Can you work these out from the model? Positions are in its coordinate system, mm. Give positions to 0.01 mm unless a question says otherwise; leave off trailing zeros. Write each loop counter-clockwise with the first axis right and the second up, starting at its lowest first coordinate (ties: lowest second). Pieces come first, ordered by that corner, then holes.
from build123d import *

# Parameters (mm, degrees)
SKETCH1_W               = 56
SKETCH1_H               = 56
SKETCH1_R               = 1.5
SKETCH1_W_2             = 46
SKETCH1_H_2             = 46
BOSS_EXTRUDE1_DEPTH     = 6
BOSS_EXTRUDE2_START     = 6
SKETCH1_2_W             = 56
SKETCH1_2_H             = 56
SKETCH1_2_R             = 1.5
BOSS_EXTRUDE2_DEPTH     = 2
CUT_EXTRUDE1_DEPTH      = 7
CUT_EXTRUDE1_DEPTH_BACK = 3
FILLET1_R               = 2


with BuildPart() as part:
    # Sketch1 → Boss-Extrude1 (new body)
    with BuildSketch(Plane(origin=(0, 0, 0), x_dir=(1, 0, 0), z_dir=(0, 1, 0))):
        Rectangle(SKETCH1_W, SKETCH1_H)
        with Locations((-25, 25)):
            Circle(SKETCH1_R, mode=Mode.SUBTRACT)
        with Locations((25, 25)):
            Circle(SKETCH1_R, mode=Mode.SUBTRACT)
        with Locations((25, -25)):
            Circle(SKETCH1_R, mode=Mode.SUBTRACT)
        with Locations((-25, -25)):
            Circle(SKETCH1_R, mode=Mode.SUBTRACT)
        Rectangle(SKETCH1_W_2, SKETCH1_H_2, mode=Mode.SUBTRACT)
    extrude(amount=BOSS_EXTRUDE1_DEPTH)

    # Sketch1<2> → Boss-Extrude2 (add)
    with BuildSketch(Plane(origin=(0, 0, 0), x_dir=(1, 0, 0), z_dir=(0, 1, 0)).offset(BOSS_EXTRUDE2_START)):
        Rectangle(SKETCH1_2_W, SKETCH1_2_H)
        with Locations((-25, 25)):
            Circle(SKETCH1_2_R, mode=Mode.SUBTRACT)
        with Locations((25, 25)):
            Circle(SKETCH1_2_R, mode=Mode.SUBTRACT)
        with Locations((25, -25)):
            Circle(SKETCH1_2_R, mode=Mode.SUBTRACT)
        with Locations((-25, -25)):
            Circle(SKETCH1_2_R, mode=Mode.SUBTRACT)
    extrude(amount=BOSS_EXTRUDE2_DEPTH)

    # Sketch2 → Cut-Extrude1 (cut, two sides)
    with BuildSketch(Plane.XZ.offset(-6)) as cut_extrude1_sk:
        Polygon((-22.732050808, 5.196152423), (-23, 4.732050808), (-23, -4.732050808), (-22.732050808, -5.196152423), (-16.732050808, -5.196152423), (-13.732050808, 0), (-16.732050808, 5.196152423), align=None)
        Polygon((-22.732050808, 16.588457268), (-23, 16.124355653), (-23, 6.660254038), (-22.732050808, 6.196152423), (-16.732050808, 6.196152423), (-13.732050808, 11.392304845), (-16.732050808, 16.588457268), align=None)
        Polygon((-3.866025404, 5.696152423), (-6.866025404, 10.892304845), (-12.866025404, 10.892304845), (-15.866025404, 5.696152423), (-12.866025404, 0.5), (-6.866025404, 0.5), align=None)
        Polygon((-12.866025404, 11.892304845), (-6.866025404, 11.892304845), (-3.866025404, 17.088457268), (-6.866025404, 22.284609691), (-12.866025404, 22.284609691), (-15.866025404, 17.088457268), align=None)
        Polygon((-6, 11.392304845), (-3, 6.196152423), (3, 6.196152423), (6, 11.392304845), (3, 16.588457268), (-3, 16.588457268), align=None)
        Polygon((6, 22.784609691), (5.875644347, 23), (-5.875644347, 23), (-6, 22.784609691), (-3, 17.588457268), (3, 17.588457268), align=None)
        Polygon((3.866025404, 17.088457268), (6.866025404, 11.892304845), (12.866025404, 11.892304845), (15.866025404, 17.088457268), (12.866025404, 22.284609691), (6.866025404, 22.284609691), align=None)
        Polygon((16.732050808, 6.196152423), (22.732050808, 6.196152423), (23, 6.660254038), (23, 16.124355653), (22.732050808, 16.588457268), (16.732050808, 16.588457268), (13.732050808, 11.392304845), align=None)
        Polygon((6.866025404, 0.5), (12.866025404, 0.5), (15.866025404, 5.696152423), (12.866025404, 10.892304845), (6.866025404, 10.892304845), (3.866025404, 5.696152423), align=None)
        Polygon((23, -4.732050808), (23, 4.732050808), (22.732050808, 5.196152423), (16.732050808, 5.196152423), (13.732050808, 0), (16.732050808, -5.196152423), (22.732050808, -5.196152423), align=None)
        Polygon((3.866025404, -5.696152423), (6.866025404, -10.892304845), (12.866025404, -10.892304845), (15.866025404, -5.696152423), (12.866025404, -0.5), (6.866025404, -0.5), align=None)
        Polygon((23, -16.124355653), (23, -6.660254038), (22.732050808, -6.196152423), (16.732050808, -6.196152423), (13.732050808, -11.392304845), (16.732050808, -16.588457268), (22.732050808, -16.588457268), align=None)
        Polygon((-6, 0), (-3, -5.196152423), (3, -5.196152423), (6, 0), (3, 5.196152423), (-3, 5.196152423), align=None)
        Polygon((-3, -6.196152423), (-6, -11.392304845), (-3, -16.588457268), (3, -16.588457268), (6, -11.392304845), (3, -6.196152423), align=None)
        Polygon((12.866025404, -11.892304845), (6.866025404, -11.892304845), (3.866025404, -17.088457268), (6.866025404, -22.284609691), (12.866025404, -22.284609691), (15.866025404, -17.088457268), align=None)
        Polygon((-5.875644347, -23), (5.875644347, -23), (6, -22.784609691), (3, -17.588457268), (-3, -17.588457268), (-6, -22.784609691), align=None)
        Polygon((-6.866025404, -0.5), (-12.866025404, -0.5), (-15.866025404, -5.696152423), (-12.866025404, -10.892304845), (-6.866025404, -10.892304845), (-3.866025404, -5.696152423), align=None)
        Polygon((-3.866025404, -17.088457268), (-6.866025404, -11.892304845), (-12.866025404, -11.892304845), (-15.866025404, -17.088457268), (-12.866025404, -22.284609691), (-6.866025404, -22.284609691), align=None)
        Polygon((-23, -6.660254038), (-23, -16.124355653), (-22.732050808, -16.588457268), (-16.732050808, -16.588457268), (-13.732050808, -11.392304845), (-16.732050808, -6.196152423), (-22.732050808, -6.196152423), align=None)
    extrude(amount=CUT_EXTRUDE1_DEPTH, mode=Mode.SUBTRACT)
    extrude(cut_extrude1_sk.sketch, amount=-CUT_EXTRUDE1_DEPTH_BACK, mode=Mode.SUBTRACT)

    # Fillet1
    fillet1_edges = [part.edges().sort_by_distance(p)[0] for p in [
        (28, 4, -28),
        (28, 4, 28),
        (-28, 4, 28),
        (-28, 4, -28),
    ]]
    fillet(fillet1_edges, radius=FILLET1_R)


solid = part.part
(1) Imagine slicing it at B-B, the plane x = -25. Write out the boundary of the cut face in (y, z).
Returned:
outline: (0, -28) - (8, -28) - (8, -26.5) - (0, -26.5) - close; (0, -23.5) - (8, -23.5) - (8, 23.5) - (0, 23.5) - close; (0, 26.5) - (8, 26.5) - (8, 28) - (0, 28) - close
(2) Imagine slicing it at A-A, the plane z = -25. Write out the boundary of the cut face in (x, y), plus the area to 3 significant figures.
Returned:
outline: (-28, 0) - (-26.5, 0) - (-26.5, 8) - (-28, 8) - close; (-23.5, 0) - (23.5, 0) - (23.5, 8) - (-23.5, 8) - close; (26.5, 0) - (28, 0) - (28, 8) - (26.5, 8) - close
area: 400 mm2
(3) Imagine slicing it at C-C, the plane y = 3.75. Write out the boundary of the cut face in (x, z), plus the area to 3 significant figures.
Returned:
outline: (-28, -26) arc R2 ccw to (-26, -28) - (26, -28) arc R2 ccw to (28, -26) - (28, 26) arc R2 ccw to (26, 28) - (-26, 28) arc R2 ccw to (-28, 26) - close; hole circle Ø3 at (-25, -25); hole circle Ø3 at (-25, 25); hole (-23, -23) - (23, -23) - (23, 23) - (-23, 23) - close; hole circle Ø3 at (25, -25); hole circle Ø3 at (25, 25)
area: 988 mm2
(4) If I drill on L1, parallel to X at y = 4, z = -25; L2, parallel to Z at x = -8.5, y = 5.25, over which ranges is the centre line in solid material (lowest first)?
Returned:
L1: x = -28 to -26.5, -23.5 to 23.5, 26.5 to 28
L2: z = -28 to -23, 23 to 28
(5) Will these pins go through, and if not, where does the flat tip stop? P1, Ø1.5, axis at x = -13, z = 11, coming from the -Y side; P2, Ø2.5, axis at x = 25, z = -25, coming from the -Y side.
Returned:
P1: stops at y = 6
P2: passes through
(6) If we mould it in two halves opening along X, with no side actions, what happens to faces 1 (the face through (-4.479, 6.986, 14.027)), 2 (the face through (-27.43, 3.94, -27.4)), 3 (the face through (27.4, 3.94, -27.43))? For each: +X half, -X half, draft (parallel to the pull), parting line (faces both ways), or undercut.
Returned:
face 1: undercut
face 2: -X half
face 3: +X half
(7) Imagine slicing it at D-D, the plane z = 10. Write out the boundary of the cut face in (x, y), plus the area to 3 significant figures.
Returned:
outline: (-28, 0) - (-23, 0) - (-23, 8) - (-28, 8) - close; (-14.54, 6) - (-13.38, 6) - (-13.38, 8) - (-14.54, 8) - close; (-6.35, 6) - (-5.2, 6) - (-5.2, 8) - (-6.35, 8) - close; (5.2, 6) - (6.35, 6) - (6.35, 8) - (5.2, 8) - close; (13.38, 6) - (14.54, 6) - (14.54, 8) - (13.38, 8) - close; (23, 0) - (28, 0) - (28, 8) - (23, 8) - close
area: 89.2 mm2
